For this review, take the finished solid that the model builds, in its own axes (mm). A direction names the side the tool comes from. Coordinates: 2 decimals unless noted, no trailing zeros. Order: outer loops, then holes, each group sorted by start corner. A loop starts at its lowest first (then second) coordinate and runs counter-clockwise, first axis right, second up.
from build123d import *

# Parameters (mm, degrees)
SKETCH_1_W      = 50
SKETCH_1_H      = 50
SKETCH_1_R      = 1.5
SKETCH_1_W_2    = 30
SKETCH_1_H_2    = 16
EXTRUDE_1_DEPTH = 2
FILLET_1_R      = 2
FILLET_2_R      = 2
FILLET_3_R      = 2
FILLET_4_R      = 2
FILLET_5_R      = 2
FILLET_6_R      = 2
FILLET_7_R      = 2
FILLET_8_R      = 2


with BuildPart() as part:
    # 草图1 → 凸台-拉伸1 (new body)
    with BuildSketch(Plane.XY):
        with Locations((4.468911917, 0.842132209)):
            Rectangle(SKETCH_1_W, SKETCH_1_H)
        with Locations((-18.031088083, 23.342132209)):
            Circle(SKETCH_1_R, mode=Mode.SUBTRACT)
        with Locations(Location((26.968911917, 23.342132209, 0), (0, 0, 180))):
            Circle(SKETCH_1_R, mode=Mode.SUBTRACT)
        with Locations((26.968911917, -21.657867791)):
            Circle(SKETCH_1_R, mode=Mode.SUBTRACT)
        with Locations(Location((-18.031088083, -21.657867791, 0), (0, 0, 180))):
            Circle(SKETCH_1_R, mode=Mode.SUBTRACT)
        with Locations((4.468911917, 0.842132209)):
            Rectangle(SKETCH_1_W_2, SKETCH_1_H_2, mode=Mode.SUBTRACT)
    extrude(amount=EXTRUDE_1_DEPTH)

    # 圆角1
    fillet_1_edges = [part.edges().sort_by_distance(p)[0] for p in [
        (19.468911917, 8.842132209, 1),
    ]]
    fillet(fillet_1_edges, radius=FILLET_1_R)

    # 圆角2
    fillet_2_edges = [part.edges().sort_by_distance(p)[0] for p in [
        (19.468911917, -7.157867791, 1),
    ]]
    fillet(fillet_2_edges, radius=FILLET_2_R)

    # 圆角3
    fillet_3_edges = [part.edges().sort_by_distance(p)[0] for p in [
        (-10.531088083, 8.842132209, 1),
    ]]
    fillet(fillet_3_edges, radius=FILLET_3_R)

    # 圆角4
    fillet_4_edges = [part.edges().sort_by_distance(p)[0] for p in [
        (-10.531088083, -7.157867791, 1),
    ]]
    fillet(fillet_4_edges, radius=FILLET_4_R)

    # 圆角5
    fillet_5_edges = [part.edges().sort_by_distance(p)[0] for p in [
        (29.468911917, 25.842132209, 1),
    ]]
    fillet(fillet_5_edges, radius=FILLET_5_R)

    # 圆角6
    fillet_6_edges = [part.edges().sort_by_distance(p)[0] for p in [
        (29.468911917, -24.157867791, 1),
    ]]
    fillet(fillet_6_edges, radius=FILLET_6_R)

    # 圆角7
    fillet_7_edges = [part.edges().sort_by_distance(p)[0] for p in [
        (-20.531088083, 25.842132209, 1),
    ]]
    fillet(fillet_7_edges, radius=FILLET_7_R)

    # 圆角8
    fillet_8_edges = [part.edges().sort_by_distance(p)[0] for p in [
        (-20.531088083, -24.157867791, 1),
    ]]
    fillet(fillet_8_edges, radius=FILLET_8_R)


solid = part.part
1. To check wall thickness, follow L1, parallel to X at y = 23.5, z = 1.95; L2, parallel to X at y = 1.5, z = 0.45; L3, parallel to Y at x = -7, z = 0.2. State the ranges of each line that lie inside material, in increasing order.
Answer below:
L1: x = -20.53 to -19.52, -16.54 to 25.48, 28.46 to 29.47
L2: x = -20.53 to -10.53, 19.47 to 29.47
L3: y = -24.16 to -7.16, 8.84 to 25.84
2. The part is to be moulded in two halves that separate along X. For faces 1 (the face through (4, -24.158, 1)), 2 (the face through (-20.531, 1, 1)), 3 (the face through (-19.137, 24.356, 0.986)), say which applies: +X half, -X half, draft (parallel to the pull), parting line (faces both ways), or undercut.
Answer below:
face 1: draft
face 2: -X half
face 3: undercut
3. Take a section at C-C, the plane z = 1.6. Give the boundary of the cut face in (x, y), plus the area to 3 significant figures.
Answer below:
outline: (-20.53, -22.16) arc R2 ccw to (-18.53, -24.16) - (27.47, -24.16) arc R2 ccw to (29.47, -22.16) - (29.47, 23.84) arc R2 ccw to (27.47, 25.84) - (-18.53, 25.84) arc R2 ccw to (-20.53, 23.84) - close; hole circle Ø3 at (-18.03, -21.66); hole circle Ø3 at (-18.03, 23.34); hole (-10.53, -5.16) arc R2 ccw to (-8.53, -7.16) - (17.47, -7.16) arc R2 ccw to (19.47, -5.16) - (19.47, 6.84) arc R2 ccw to (17.47, 8.84) - (-8.53, 8.84) arc R2 ccw to (-10.53, 6.84) - close; hole circle Ø3 at (26.97, -21.66); hole circle Ø3 at (26.97, 23.34)
area: 1,990 mm2
4. Take a section at A-A, the plane y = 2. Give the boundary of the cut face in (x, z), plus the area to 3 significant figures.
Answer below:
outline: (-20.53, 0) - (-10.53, 0) - (-10.53, 2) - (-20.53, 2) - close; (19.47, 0) - (29.47, 0) - (29.47, 2) - (19.47, 2) - close
area: 40.0 mm2
5. Machinability: for faces 4 (the face through (-9.96, -6.56, 1.01)), 5 (the face through (-19.9, 25.3, 1)), which of the approach directions +Z, -Z, +X, -X, +Y, -Y give a long, thin tool a straight path to every point of the face, cutting with its end or side? Answer none if there is none.
Answer below:
face 4: +Z, -Z
face 5: +Z, -Z, -X, +Y
6. Take a section at B-B, the plane x = 15. Give the boundary of the cut face in (y, z).
Answer below:
outline: (-24.16, 0) - (-7.16, 0) - (-7.16, 2) - (-24.16, 2) - close; (8.84, 0) - (25.84, 0) - (25.84, 2) - (8.84, 2) - close
